from build123d import *

# Parameters (mm, degrees)
BOSS_EXTRUDE1_DEPTH  = 3.2
SKETCH2_R            = 2.4
BOSS_EXTRUDE2_DEPTH  = 1.6
LPATTERN1_COUNT      = 12
LPATTERN1_PITCH      = 8
LPATTERN1_COUNT_DIR2 = 3
LPATTERN1_PITCH_DIR2 = 8
SKETCH3_R            = 2.4
BOSS_EXTRUDE3_DEPTH  = 1.6
LPATTERN2_COUNT      = 9
LPATTERN2_PITCH      = 8
SKETCH4_R            = 2.4
BOSS_EXTRUDE4_DEPTH  = 1.6
LPATTERN3_COUNT      = 6
LPATTERN3_PITCH      = 8
SKETCH5_R            = 2.4
BOSS_EXTRUDE5_DEPTH  = 1.6
LPATTERN4_COUNT      = 3
LPATTERN4_PITCH      = 8
SHELL1_T             = -1.6


with BuildPart() as part:
    # Sketch1 → Boss-Extrude1 (new body)
    with BuildSketch(Plane(origin=(0, 0, 0), x_dir=(1, 0, 0), z_dir=(0, 1, 0))):
        Polygon((0, 0), (96, 0), (96, -24), (24, -48), (0, -48), align=None)
    extrude(amount=BOSS_EXTRUDE1_DEPTH)

    # Sketch2 → Boss-Extrude2 (add)
    with BuildSketch(Plane(origin=(0, 3.2, 0), x_dir=(1, 0, 0), z_dir=(0, 1, 0))):
        with Locations(Location((4, -4, 0), (0, 0, 90))):
            Circle(SKETCH2_R)
    boss_extrude2 = extrude(amount=BOSS_EXTRUDE2_DEPTH)

    # LPattern1: Boss-Extrude2 12 × 3
    with Locations(*[(i * LPATTERN1_PITCH, 0, j * LPATTERN1_PITCH_DIR2) for i in range(LPATTERN1_COUNT) for j in range(LPATTERN1_COUNT_DIR2) if (i, j) != (0, 0)]):
        add(boss_extrude2)

    # Sketch3 → Boss-Extrude3 (add)
    with BuildSketch(Plane(origin=(0, 3.2, 0), x_dir=(1, 0, 0), z_dir=(0, 1, 0))):
        with Locations(Location((4, -28, 0), (0, 0, 90))):
            Circle(SKETCH3_R)
    boss_extrude3 = extrude(amount=BOSS_EXTRUDE3_DEPTH)

    # LPattern2: Boss-Extrude3 ×9
    with Locations(*[(i * LPATTERN2_PITCH, 0, 0) for i in range(1, LPATTERN2_COUNT)]):
        add(boss_extrude3)

    # Sketch4 → Boss-Extrude4 (add)
    with BuildSketch(Plane(origin=(0, 3.2, 0), x_dir=(1, 0, 0), z_dir=(0, 1, 0))):
        with Locations(Location((4, -36, 0), (0, 0, 90))):
            Circle(SKETCH4_R)
    boss_extrude4 = extrude(amount=BOSS_EXTRUDE4_DEPTH)

    # LPattern3: Boss-Extrude4 ×6
    with Locations(*[(i * LPATTERN3_PITCH, 0, 0) for i in range(1, LPATTERN3_COUNT)]):
        add(boss_extrude4)

    # Sketch5 → Boss-Extrude5 (add)
    with BuildSketch(Plane(origin=(0, 3.2, 0), x_dir=(1, 0, 0), z_dir=(0, 1, 0))):
        with Locations(Location((4, -44, 0), (0, 0, 90))):
            Circle(SKETCH5_R)
    boss_extrude5 = extrude(amount=BOSS_EXTRUDE5_DEPTH)

    # LPattern4: Boss-Extrude5 ×3
    with Locations(*[(i * LPATTERN4_PITCH, 0, 0) for i in range(1, LPATTERN4_COUNT)]):
        add(boss_extrude5)

    # Shell1
    shell1_openings = [part.faces().sort_by_distance(p)[0] for p in [
        (42.461538462, 0, 20.307692308),
    ]]
    offset(amount=SHELL1_T, openings=shell1_openings, kind=Kind.INTERSECTION)


solid = part.part
Read the model definition and answer for the solid it produces. Units are mm, in the model's axes. A direction names the side the tool comes from. Give positions to 0.01 mm unless a question says otherwise; leave off trailing zeros. Write each loop counter-clockwise with the first axis right and the second up, starting at its lowest first coordinate (ties: lowest second). Pieces come first, ordered by that corner, then holes. Notation, with made-up numbers: (32.5, 49) - (87.5, 49) arc R14 ccw to (87.5, 57) - close; hole circle Ø1 at (-36, 62). An arc over 180 degrees is marked (long way). Use CSV: the item, a comma, the result in double quotes. Start each with the question number.
(1) Consider line 1 along Z through (x, y) = (11.5, 1.1); line 2 along Z through (x, y) = (84, 2.95); line 3 along Y through (x, z) = (16.5, 22). Determine where each line is inside the solid, lowest interval first.
(2) For faces 3 (the flat face through (59.56, 0.79, 34.46)), 4 (the flat face through (52, 4.8, 20)), 5 (the cylindrical face through (46.343, 3.989, 28.52)), determine the directions among +Z, -Z, +X, -X, +Y, -Y from which every point of the face is accessible in a straight line to the end or side of a thin tool.
(3) Determine the mould class of faces 1 (the flat face through (66, 0, 33)), 2 (the cylindrical face through (21.46, 3.989, 29.905)) for opening direction X: +X half, -X half, draft (parallel to the pull), parting line (faces both ways), or undercut.
(4) Find section A-A (y = 0.8). Give the vertices of the cut face in (x, z).
(5) Find section B-B (x = 7.5). Give the vertices of the cut face in (y, z), plus the area to 3 significant figures.
(6) Given P1, Ø2, axis at x = 32, z = 20.5, coming from the +Y side; P2, Ø0.5, axis at x = 20.5, z = 20, coming from the -Y side; P3, Ø1.5, axis at y = 4, z = 42.5, coming from the +X side; P4, Ø10, axis at x = 11, z = 17, coming from the +Y side, each flat-ended and moving along its own axis, determine where each tip first touches the part or whether it passes through.
Findings below:
1,line 1,"0 to 1.6, 46.4 to 48"
1,line 2,"0 to 3.2, 4.8 to 11.2, 12.8 to 19.2, 20.8 to 28"
1,line 3,"1.6 to 3.2"
2,face 3,"-Y"
2,face 4,"+Z, -Z, +X, -X, +Y"
2,face 5,"+Y"
3,face 1,"draft"
3,face 2,"undercut"
4,outline,"(0, 0) - (96, 0) - (96, 24) - (24, 48) - (0, 48) - close; hole (1.6, 1.6) - (94.4, 1.6) - (94.4, 22.85) - (23.74, 46.4) - (1.6, 46.4) - close"
5,outline,"(0, 0) - (3.2, 0) - (3.2, 48) - (0, 48) - (0, 46.4) - (1.6, 46.4) - (1.6, 1.6) - (0, 1.6) - close"
5,area,"81.9 mm2"
6,P1,"y = 3.2"
6,P2,"y = 3.2"
6,P3,"x = 22.28"
6,P4,"y = 4.8"
